from build123d import *
from OCP.BRepFilletAPI import BRepFilletAPI_MakeChamfer

# Parameters (mm, degrees)
CROQUIS1_R              = 1.549999999999994
CROQUIS1_R_2            = 2.5499999999999923
CROQUIS1_R_3            = 2.5500000000020107
CROQUIS1_R_4            = 2.5499999999987524
CROQUIS1_R_5            = 1.5500000000000012
SALIENTE_EXTRUIR1_DEPTH = 5
REDONDEO1_R             = 10
REDONDEO2_R             = 10
REDONDEO4_R             = 2.5
CHAFL_N1_SIZE           = 50
CHAFL_N1_SIZE2          = 25
CROQUIS2_R              = 2.5499999999999914
SALIENTE_EXTRUIR2_DEPTH = 5
REDONDEO5_R             = 25


with BuildPart() as part:
    # Croquis1 → Saliente-Extruir1 (new body)
    with BuildSketch(Plane.XY):
        with BuildLine():
            Line((22.499999999999602, 23.448771432804598), (22.499999999999606, 10.00000000000557))
            Line((22.499999999999606, 10.00000000000557), (28.23305122348206, 10.00000000000557))
            Line((28.23305122348206, 10.00000000000557), (28.233051223482065, -9.999999999994426))
            Line((28.233051223482065, -9.999999999994426), (22.49999999999961, -9.99999999999443))
            Line((22.49999999999961, -9.99999999999443), (22.49999999999961, -20.499999999994426))
            Line((22.49999999999961, -20.499999999994426), (22.49999999999961, -23.448771432804598))
            Line((22.49999999999961, -23.448771432804598), (15.3999999999996, -23.448771432804598))
            ThreePointArc((15.3999999999996, -23.448771432804598), (3.787647475656714, -38.722635385727685), (21.610549895016423, -45.827689963420795))
            Line((21.610549895016423, -45.827689963420795), (23.615707001015654, -44.64130534237437))
            Line((23.615707001015654, -44.64130534237437), (79.74064487017472, -11.416377836244111))
            Line((79.74064487017472, -11.416377836244111), (82.13324958071296, -10))
            Line((82.13324958071296, -10), (182.8500644459697, -9.999999999999998))
            Line((182.8500644459697, -9.999999999999998), (182.8500644459697, 9.999999999999998))
            Line((182.8500644459697, 9.999999999999998), (87.50000000000001, 9.999999999999998))
            Line((87.50000000000001, 9.999999999999998), (82.13324958071296, 9.999999999999998))
            Line((82.13324958071296, 9.999999999999998), (23.615707001015654, 44.64130534237437))
            Line((23.615707001015654, 44.64130534237437), (21.610549895016423, 45.827689963420795))
            ThreePointArc((21.610549895016423, 45.827689963420795), (3.787647475656714, 38.722635385727685), (15.3999999999996, 23.448771432804598))
            Line((15.3999999999996, 23.448771432804598), (22.499999999999602, 23.448771432804598))
        make_face()
        with Locations((170.68634124367938, 0)):
            Circle(CROQUIS1_R, mode=Mode.SUBTRACT)
        with Locations((75.6, 0)):
            Circle(CROQUIS1_R_2, mode=Mode.SUBTRACT)
        with Locations((15.3999999999996, -35.50000000000558)):
            Circle(CROQUIS1_R_3, mode=Mode.SUBTRACT)
        with Locations((15.3999999999996, 35.50000000000558)):
            Circle(CROQUIS1_R_4, mode=Mode.SUBTRACT)
        with Locations((95.6863412436794, 0)):
            Circle(CROQUIS1_R, mode=Mode.SUBTRACT)
        with Locations((145.68634124367938, 0)):
            Circle(CROQUIS1_R, mode=Mode.SUBTRACT)
        with Locations((120.68634124367938, 0)):
            Circle(CROQUIS1_R, mode=Mode.SUBTRACT)
        with Locations((38.875017115898416, 0)):
            Circle(CROQUIS1_R_5, mode=Mode.SUBTRACT)
        with Locations((58.875017115898416, -1.73e-15)):
            Circle(CROQUIS1_R_5, mode=Mode.SUBTRACT)
    extrude(amount=SALIENTE_EXTRUIR1_DEPTH)

    # Redondeo1
    redondeo1_edges = [part.edges().sort_by_distance(p)[0] for p in [
        (22.49999999999961, -23.448771432804598, 2.5),
        (22.499999999999602, 23.448771432804598, 2.5),
    ]]
    fillet(redondeo1_edges, radius=REDONDEO1_R)

    # Redondeo2
    redondeo2_edges = [part.edges().sort_by_distance(p)[0] for p in [
        (182.8500644459697, -9.999999999999998, 2.5),
        (182.8500644459697, 9.999999999999998, 2.5),
    ]]
    fillet(redondeo2_edges, radius=REDONDEO2_R - 0.0001)  # a hair under: the kernel refuses the full size

    # Redondeo4
    redondeo4_edges = [part.edges().sort_by_distance(p)[0] for p in [
        (22.49999999999961, -9.99999999999443, 2.5),
        (28.233051223482065, -9.999999999994426, 2.5),
        (28.23305122348206, 10.00000000000557, 2.5),
        (22.499999999999606, 10.00000000000557, 2.5),
    ]]
    fillet(redondeo4_edges, radius=REDONDEO4_R)

    # Chaflán1: one chamfer whose edges measure the first distance from different faces: ONE call of the kernel's chamfer builder (chamfer() names one face for all edges)
    chafl_n1_edges_1 = [part.edges().sort_by_distance(p)[0] for p in [
        (82.13324958071296, 9.999999999999998, 2.5),
    ]]
    chafl_n1_side_1 = [part.faces().sort_by_distance(p)[0] for p in [
        (127.49170701334134, 9.999999999999998, 2.5),
    ]]
    chafl_n1_edges_2 = [part.edges().sort_by_distance(p)[0] for p in [
        (82.13324958071296, -10, 2.5),
    ]]
    chafl_n1_side_2 = [part.faces().sort_by_distance(p)[0] for p in [
        (52.874478290864296, -27.320652671187155, 2.5),
    ]]
    chafl_n1 = BRepFilletAPI_MakeChamfer(part.part.solid().wrapped)
    for e in chafl_n1_edges_1:
        chafl_n1.Add(CHAFL_N1_SIZE, CHAFL_N1_SIZE2, e.wrapped, chafl_n1_side_1[0].wrapped)  # the first distance lies on this face
    for e in chafl_n1_edges_2:
        chafl_n1.Add(CHAFL_N1_SIZE, CHAFL_N1_SIZE2, e.wrapped, chafl_n1_side_2[0].wrapped)  # the first distance lies on this face
    add(Compound.cast(chafl_n1.Shape()), mode=Mode.REPLACE)

    # Croquis2 → Saliente-Extruir2 (add)
    with BuildSketch(Plane(origin=(0, 0, 0), x_dir=(-1, 0, 0), z_dir=(0, 0, -1))):
        with BuildLine():
            Line((-96.37672384904373, 16.36766473551684), (-82.582860744419, 37.547706950275206))
            ThreePointArc((-82.582860744419, 37.547706950275206), (-79.57146676248833, 40.32594256297316), (-75.59999999999961, 41.33318562624969))
            Line((-75.59999999999961, 41.33318562624969), (-15.399999999999643, 47.55122856720654))
            Line((-15.399999999999643, 47.55122856720654), (-60.62019811737546, 22.735329471033683))
            Line((-60.62019811737546, 22.735329471033683), (-96.37672384904373, 16.36766473551684))
        make_face()
        with Locations((-75.59999999999961, 33)):
            Circle(CROQUIS2_R, mode=Mode.SUBTRACT)
    extrude(amount=-SALIENTE_EXTRUIR2_DEPTH)

    # Redondeo5
    redondeo5_edges = [part.edges().sort_by_distance(p)[0] for p in [
        (96.37672384904373, 16.36766473551684, 2.5),
    ]]
    fillet(redondeo5_edges, radius=REDONDEO5_R)


solid = part.part
Here's how the part is built. I have some questions about the finished solid (model axes, mm). A direction names the side the tool comes from. Coordinates: 2 decimals unless noted, no trailing zeros. Order: outer loops, then holes, each group sorted by start corner. A loop starts at its lowest first (then second) coordinate and runs counter-clockwise, first axis right, second up. Notation, with made-up numbers: (60.25, 66) -> (75.25, 66) arc R19 ccw to (75.25, 70) -> close; hole circle Ø8 at (12, 59). An arc over 180 degrees is marked (long way). Answer in a Markdown table with one row per item.
(1) On a 3-axis mill with a long thin cutter (end or side, diameter ignored), from which of +Z, -Z, +X, -X, +Y, -Y can I reach the whole of each face in a straight line? I mean faces 1 (the face through (153, 10, 2)), 2 (the face through (28.233, 0, 2)), 3 (the face through (37.327, 0.068, 2.465)). Say none if no direction works.
Answer key:
| item | result |
|---|---|
| face 1 | +Z, -Z, +X, +Y |
| face 2 | +Z, -Z, -X |
| face 3 | +Z, -Z |
(2) Thinking about a two-plate mould opening in Y: for faces 4 (the face through (180, -6.99, 2.54)), 5 (the face through (14.85, -37.99, 2.46)), 6 (the face through (72, 1, 0)), 7 (the face through (73.052, 0.112, 2.465)), which applies, +Y half, -Y half, draft (parallel to the pull), parting line (faces both ways), or undercut?
Answer key:
| item | result |
|---|---|
| face 4 | -Y half |
| face 5 | undercut |
| face 6 | draft |
| face 7 | undercut |
(3) Will these pins go through, and if not, where does the flat tip stop? pin 1 Ø1.5 at (y, z) = (-3, 1.5) entering from -X; pin 2 Ø2.5 at (x, z) = (127.5, 3) entering from -Y; pin 3 Ø3.5 at (x, y) = (95.69, 0) entering from -Z; pin 4 Ø3 at (y, z) = (9, 0.5) entering from -X.
Answer key:
| item | result |
|---|---|
| pin 1 | x = 28.23 |
| pin 2 | y = -10 |
| pin 3 | z = 0 |
| pin 4 | x = 23.5 |
(4) I want a section at A-A on z = 3.95. Count the separate pieces of the cut face and the enclosed holes in it, then the cut area to 3 significant figures.
Answer key:
| item | result |
|---|---|
| separate pieces | 1 |
| enclosed holes | 10 |
| area | 7,510 mm^2 |
(5) I want a section at C-C on x = 113.5. List the corners of the cut face in (y, z) for me, then the cut area to 3 significant figures.
Answer key:
| item | result |
|---|---|
| outline | (-10, 0) -> (13.32, 0) -> (13.32, 5) -> (-10, 5) -> close |
| area | 117 mm^2 |
(6) I want a section at B-B on y = -41.5. List the corners of the cut face in (x, z) for me.
Answer key:
| item | result |
|---|---|
| outline | (4.95, 0) -> (28.92, 0) -> (28.92, 5) -> (4.95, 5) -> close |
(7) Please list where these lines run through material, in increasing order: probe 1 along Y at (x, z) = (136.5, 0.4); probe 2 along Y at (x, z) = (75.6, 3.95); probe 3 along Y at (x, z) = (28, 1).
Answer key:
| item | result |
|---|---|
| probe 1 | -10 to 10 |
| probe 2 | -21.81 to -2.55, 2.55 to 30.45, 35.55 to 41.33 |
| probe 3 | -42.05 to -8.55, 8.55 to 46.25 |
